Work out the finished part from the listing and answer in its coordinate system (mm). A direction names the side the tool comes from. Give positions to 0.01 mm unless a question says otherwise; leave off trailing zeros. Write each loop counter-clockwise with the first axis right and the second up, starting at its lowest first coordinate (ties: lowest second). Pieces come first, ordered by that corner, then holes. Notation, with made-up numbers: (23.25, 22.25) -> (77.25, 22.25) arc R17 ccw to (77.25, 30.25) -> close; hole circle Ø8 at (27, -23.75). An arc over 180 degrees is marked (long way). Use a Markdown table: item, result. Add a question column.
Q1. Section B-B, the plane x = -2 is taken. Give the vertices of the cut face in (y, z).
Q2. For faces 5 (the face through (9, -31, 1)), 6 (the face through (-9, 31, 1)), 7 (the face through (0, -3.25, 1)), 8 (the face through (-21.5, -13, 1)), 9 (the face through (21.5, -13, 1)), determine the directions among +Z, -Z, +X, -X, +Y, -Y from which every point of the face is accessible in a straight line to the end or side of a thin tool.
Q3. Consider line 1 (Y direction, x = 18, z = 0.4); line 2 (Y direction, x = -15.25, z = 1.45); line 3 (X direction, y = -14, z = 0.9). Determine where each line is inside the solid, lowest interval first.
Q4. Section C-C, the plane z = 0.95 is taken. State how many separate pieces and enclosed holes the cut face has, plus the area to 3 significant figures.
Q5. For a pull along X with two mould halves and no side action, classify faces 1 (the face through (7.4, 2.68, 0.99)), 2 (the face through (-23, 31, 1)), 3 (the face through (17, 0, 1)), 4 (the face through (19, 10.25, 1)) as pulls with the +X half, pulls with the -X half, needs draft (parallel to the pull), parting line crosses it, or undercut.
Q6. Section A-A, the plane y = -15.25 is taken. Give the vertices of the cut face in (x, z), plus the area to 3 significant figures.
Q7. Each of these flat-tipped pins is pushed along its axis until it touches: pin 1 Ø1 at (y, z) = (0.5, 1.5) entering from -X; pin 2 Ø4.5 at (x, y) = (-18, -25) entering from +Z; pin 3 Ø3 at (x, y) = (15.25, 15.25) entering from +Z; pin 4 Ø1 at (y, z) = (-12.5, 0.5) entering from +X. Where does it stop, or does it pass through?
from build123d import *

# Parameters (mm, degrees)
F0_R     = 1.75
F1_DEPTH = 2
F2_R     = 5


with BuildPart() as f1:
    # F0 (on Top) → F1 (new body)
    with BuildSketch(Plane.XY):
        with BuildLine():
            Line((-13, 41), (-18, 41))
            ThreePointArc((-18, 41), (-21.5355339059, 39.5355339059), (-23, 36))
            Line((-23, 36), (-23, 25.7647321898))
            ThreePointArc((-23, 25.7647321898), (-22.9708868654, 25.0022263751), (-22.8837169765, 24.2441603473))
            Line((-22.8837169765, 24.2441603473), (-21.6162830235, 16.0058396527))
            ThreePointArc((-21.6162830235, 16.0058396527), (-21.5291131346, 15.2477736249), (-21.5, 14.4852678102))
            Line((-21.5, 14.4852678102), (-21.5, 11.25))
            ThreePointArc((-21.5, 11.25), (-21.2071067812, 10.5428932188), (-20.5, 10.25))
            Line((-20.5, 10.25), (-18, 10.25))
            ThreePointArc((-18, 10.25), (-17.2928932188, 9.9571067812), (-17, 9.25))
            Line((-17, 9.25), (-17, -9.25))
            ThreePointArc((-17, -9.25), (-17.2928932188, -9.9571067812), (-18, -10.25))
            Line((-18, -10.25), (-20.5, -10.25))
            ThreePointArc((-20.5, -10.25), (-21.2071067812, -10.5428932188), (-21.5, -11.25))
            Line((-21.5, -11.25), (-21.5, -14.4852678102))
            ThreePointArc((-21.5, -14.4852678102), (-21.5291131346, -15.2477736249), (-21.6162830235, -16.0058396527))
            Line((-21.6162830235, -16.0058396527), (-22.8837169765, -24.2441603473))
            ThreePointArc((-22.8837169765, -24.2441603473), (-22.9708868654, -25.0022263751), (-23, -25.7647321898))
            Line((-23, -25.7647321898), (-23, -36))
            ThreePointArc((-23, -36), (-21.5355339059, -39.5355339059), (-18, -41))
            Line((-18, -41), (-13, -41))
            Line((-13, -41), (-13, -39))
            ThreePointArc((-13, -39), (-10.0710678119, -31.9289321881), (-3, -29))
            Line((-3, -29), (0, -29))
            Line((0, -29), (3, -29))
            ThreePointArc((3, -29), (10.0710678119, -31.9289321881), (13, -39))
            Line((13, -39), (13, -41))
            Line((13, -41), (18, -41))
            ThreePointArc((18, -41), (21.5355339059, -39.5355339059), (23, -36))
            Line((23, -36), (23, -25.7647321898))
            ThreePointArc((23, -25.7647321898), (22.9708868654, -25.0022263751), (22.8837169765, -24.2441603473))
            Line((22.8837169765, -24.2441603473), (21.6162830235, -16.0058396527))
            ThreePointArc((21.6162830235, -16.0058396527), (21.5291131346, -15.2477736249), (21.5, -14.4852678102))
            Line((21.5, -14.4852678102), (21.5, -11.25))
            ThreePointArc((21.5, -11.25), (21.2071067812, -10.5428932188), (20.5, -10.25))
            Line((20.5, -10.25), (18, -10.25))
            ThreePointArc((18, -10.25), (17.2928932188, -9.9571067812), (17, -9.25))
            Line((17, -9.25), (17, 9.25))
            ThreePointArc((17, 9.25), (17.2928932188, 9.9571067812), (18, 10.25))
            Line((18, 10.25), (20.5, 10.25))
            ThreePointArc((20.5, 10.25), (21.2071067812, 10.5428932188), (21.5, 11.25))
            Line((21.5, 11.25), (21.5, 14.4852678102))
            ThreePointArc((21.5, 14.4852678102), (21.5291131346, 15.2477736249), (21.6162830235, 16.0058396527))
            Line((21.6162830235, 16.0058396527), (22.8837169765, 24.2441603473))
            ThreePointArc((22.8837169765, 24.2441603473), (22.9708868654, 25.0022263751), (23, 25.7647321898))
            Line((23, 25.7647321898), (23, 36))
            ThreePointArc((23, 36), (21.5355339059, 39.5355339059), (18, 41))
            Line((18, 41), (13, 41))
            Line((13, 41), (13, 39))
            ThreePointArc((13, 39), (10.0710678119, 31.9289321881), (3, 29))
            Line((3, 29), (0, 29))
            Line((0, 29), (-3, 29))
            ThreePointArc((-3, 29), (-10.0710678119, 31.9289321881), (-13, 39))
            Line((-13, 39), (-13, 41))
        make_face()
        with Locations((-18, -36)):
            Circle(F0_R, mode=Mode.SUBTRACT)
        with Locations((-18, -25)):
            Circle(F0_R, mode=Mode.SUBTRACT)
        with Locations((-15.25, -15.25)):
            Circle(F0_R, mode=Mode.SUBTRACT)
        with Locations((18, -36)):
            Circle(F0_R, mode=Mode.SUBTRACT)
        with Locations((18, -25)):
            Circle(F0_R, mode=Mode.SUBTRACT)
        with BuildLine():
            Line((6, -13), (-6, -13))
            ThreePointArc((-6, -13), (-7.4142135624, -12.4142135624), (-8, -11))
            Line((-8, -11), (-8, -8.5))
            ThreePointArc((-8, -8.5), (-7.4142135624, -7.0857864376), (-6, -6.5))
            Line((-6, -6.5), (6, -6.5))
            ThreePointArc((6, -6.5), (7.4142135624, -7.0857864376), (8, -8.5))
            Line((8, -8.5), (8, -11))
            ThreePointArc((8, -11), (7.4142135624, -12.4142135624), (6, -13))
        make_face(mode=Mode.SUBTRACT)
        with Locations((15.25, -15.25)):
            Circle(F0_R, mode=Mode.SUBTRACT)
        with Locations((-15.25, 15.25)):
            Circle(F0_R, mode=Mode.SUBTRACT)
        with Locations((-18, 25)):
            Circle(F0_R, mode=Mode.SUBTRACT)
        with Locations((-18, 36)):
            Circle(F0_R, mode=Mode.SUBTRACT)
        with BuildLine():
            ThreePointArc((-8, 1.25), (-7.4142135624, 2.6642135624), (-6, 3.25))
            Line((-6, 3.25), (6, 3.25))
            ThreePointArc((6, 3.25), (7.4142135624, 2.6642135624), (8, 1.25))
            Line((8, 1.25), (8, -1.25))
            ThreePointArc((8, -1.25), (7.4142135624, -2.6642135624), (6, -3.25))
            Line((6, -3.25), (-6, -3.25))
            ThreePointArc((-6, -3.25), (-7.4142135624, -2.6642135624), (-8, -1.25))
            Line((-8, -1.25), (-8, 1.25))
        make_face(mode=Mode.SUBTRACT)
        with BuildLine():
            ThreePointArc((-8, 11), (-7.4142135624, 12.4142135624), (-6, 13))
            Line((-6, 13), (6, 13))
            ThreePointArc((6, 13), (7.4142135624, 12.4142135624), (8, 11))
            Line((8, 11), (8, 8.5))
            ThreePointArc((8, 8.5), (7.4142135624, 7.0857864376), (6, 6.5))
            Line((6, 6.5), (-6, 6.5))
            ThreePointArc((-6, 6.5), (-7.4142135624, 7.0857864376), (-8, 8.5))
            Line((-8, 8.5), (-8, 11))
        make_face(mode=Mode.SUBTRACT)
        with Locations((15.25, 15.25)):
            Circle(F0_R, mode=Mode.SUBTRACT)
        with Locations((18, 25)):
            Circle(F0_R, mode=Mode.SUBTRACT)
        with Locations((18, 36)):
            Circle(F0_R, mode=Mode.SUBTRACT)
    extrude(amount=F1_DEPTH)

    # F2
    f2_edges = [f1.edges().sort_by_distance(p)[0] for p in [
        (-13, -41, 1),
        (13, -41, 1),
        (-13, 41, 1),
        (13, 41, 1),
    ]]
    fillet(f2_edges, radius=F2_R)


solid = f1.part
Result set:
| question | item | result |
|---|---|---|
| 1 | outline | (-29, 0) -> (-13, 0) -> (-13, 2) -> (-29, 2) -> close; (-6.5, 0) -> (-3.25, 0) -> (-3.25, 2) -> (-6.5, 2) -> close; (3.25, 0) -> (6.5, 0) -> (6.5, 2) -> (3.25, 2) -> close; (13, 0) -> (29, 0) -> (29, 2) -> (13, 2) -> close |
| 2 | face 5 | +Z, -Z, -Y |
| 2 | face 6 | +Z, -Z, +Y |
| 2 | face 7 | +Z, -Z |
| 2 | face 8 | +Z, -Z, -X |
| 2 | face 9 | +Z, -Z, +X |
| 3 | line 1 | y = -41 to -37.75, -34.25 to -26.75, -23.25 to -10.25, 10.25 to 23.25, 26.75 to 34.25, 37.75 to 41 |
| 3 | line 2 | y = -40.36 to -17, -13.5 to 13.5, 17 to 40.36 |
| 3 | line 3 | x = -21.5 to -16.47, -14.03 to 14.03, 16.47 to 21.5 |
| 4 | separate pieces | 1 |
| 4 | enclosed holes | 15 |
| 4 | area | 2,470 mm2 |
| 5 | face 1 | undercut |
| 5 | face 2 | pulls with the -X half |
| 5 | face 3 | pulls with the +X half |
| 5 | face 4 | needs draft |
| 6 | outline | (-21.53, 0) -> (-17, 0) -> (-17, 2) -> (-21.53, 2) -> close; (-13.5, 0) -> (13.5, 0) -> (13.5, 2) -> (-13.5, 2) -> close; (17, 0) -> (21.53, 0) -> (21.53, 2) -> (17, 2) -> close |
| 6 | area | 72.1 mm2 |
| 7 | pin 1 | stops at x = -17 |
| 7 | pin 2 | stops at z = 2 |
| 7 | pin 3 | passes through |
| 7 | pin 4 | stops at x = 21.5 |
